Autodesk Inventor part; units mm, degrees
ref_plane "YZ Plane" through (0, 0, 0) normal (1, 0, 0) x (0, 1, 0)
ref_plane "XZ Plane" through (0, 0, 0) normal (0, 1, 0) x (-1, 0, 0)
ref_plane "XY Plane" through (0, 0, 0) normal (0, 0, 1) x (1, 0, 0)
sketch "스케치1" plane through (0, 0, 0) normal (0, 1, 0) x (-1, 0, 0)
  line L0 (-9.4, 28.75) -> (9.4, 28.75)
  line L1 (9.4, 28.75) -> (9.4, -28.75)
  line L2 (9.4, -28.75) -> (-9.4, -28.75)
  line L3 (-9.4, -28.75) -> (-9.4, 28.75)
  line L4 (-9.4, 28.75) -> (9.4, -28.75) construction
  line L5 (9.4, 28.75) -> (-9.4, -28.75) construction
  line L6 (-11.4, -30.75) -> (11.4, -30.75)
  line L7 (11.4, -30.75) -> (11.4, 30.75)
  line L8 (11.4, 30.75) -> (-11.4, 30.75)
  line L9 (-11.4, 30.75) -> (-11.4, -30.75)
  point P0 (0, 0)
  dimension "d0" = 18.8
  dimension "d1" = 57.5
  dimension "d2" = 2
extrude "돌출1" add sketch "스케치1" against normal blind 2 contours L0 L1 L2 L3
extrude "돌출2" add sketch "스케치1" against normal blind 6
sketch "스케치2" plane through (0, -6, 0) normal (0, -1, 0) x (1, 0, 0)
  line L0 (11.4, -30.75) -> (11.4, 30.75)
  line L1 (9.4, 28.75) -> (9.4, -28.75)
  line L2 (9.4, -28.75) -> (-9.4, -28.75)
  line L3 (11.4, -28.75) -> (9.1, -28.75)
  line L4 (9.1, -28.75) -> (9.1, -23.75)
  line L5 (9.1, -23.75) -> (11.4, -23.75)
  line L6 (11.4, -23.75) -> (11.4, -28.75)
  line L7 (0, 0) -> (0, -17.1125) construction
  line L8 (0, 0) -> (-6.0193, 0) construction
  line L9 (-11.4, -28.75) -> (-9.1, -28.75)
  line L10 (-9.1, -28.75) -> (-9.1, -23.75)
  line L11 (-9.1, -23.75) -> (-11.4, -23.75)
  line L12 (11.4, 28.75) -> (9.1, 28.75)
  line L13 (9.1, 28.75) -> (9.1, 23.75)
  line L14 (9.1, 23.75) -> (11.4, 23.75)
  line L15 (-9.1, 28.75) -> (-9.1, 23.75)
  line L16 (-11.4, 28.75) -> (-9.1, 28.75)
  line L17 (-9.1, 23.75) -> (-11.4, 23.75)
  line L18 (-11.4, 30.75) -> (-11.4, -30.75)
  line L19 (-11.4, -28.75) -> (-11.4, -23.75)
  line L20 (-11.4, 23.75) -> (-11.4, 28.75)
  line L21 (11.4, 23.75) -> (11.4, 28.75)
  point P0 (-9.1, -28.75)
  dimension "d7" = 0.3
  dimension "d8" = 5
extrude "돌출3" add sketch "스케치2" along normal blind 2 contours L3 L1 L5 L0 | L18 L16 L15 L17 | L2 L9 L18 L11 L10 | L2 L4 L5 L1 | L14 L1 L12 L0 | L14 L13 L12 L1
sketch "스케치3" plane through (0, 0, 0) normal (0, 1, 0) x (1, 0, 0)
  line L0 (6.25, -23) -> (-6.25, -23)
  line L1 (-6.25, -23) -> (-6.25, 23)
  line L2 (-6.25, 23) -> (6.25, 23)
  line L3 (6.25, 23) -> (6.25, -23)
  line L4 (6.25, -23) -> (-6.25, 23) construction
  line L5 (-6.25, -23) -> (6.25, 23) construction
  line L6 (0, -23) -> (0, 23) construction
  line L7 (9.4, -23.75) -> (9.4, 23.75) construction
  line L8 (9.4, 0) -> (-6.25, 0) construction
  line L9 (-6.25, -23) -> (-9.25, -23)
  line L10 (-9.25, -23) -> (-9.25, -13)
  line L11 (-9.25, -13) -> (-6.25, -13)
  line L12 (-6.25, -13) -> (-6.25, -23)
  line L13 (6.25, -23) -> (9.25, -23)
  line L14 (9.25, -23) -> (9.25, -13)
  line L15 (9.25, -13) -> (6.25, -13)
  line L16 (6.25, -13) -> (6.25, -23)
  line L17 (-6.25, 23) -> (-9.25, 23)
  line L18 (-9.25, 23) -> (-9.25, 13)
  line L19 (-9.25, 13) -> (-6.25, 13)
  line L20 (-6.25, 13) -> (-6.25, 23)
  line L21 (9.25, 13) -> (6.25, 13)
  line L22 (6.25, 13) -> (6.25, 23)
  line L23 (9.25, 23) -> (9.25, 13)
  line L24 (6.25, 23) -> (9.25, 23)
  point P0 (0, 0)
  dimension "d12" = 46
  dimension "d13" = 3
  dimension "d14" = 10
  dimension "d15" = 9.25
extrude "돌출4" add sketch "스케치3" along normal blind 5 contours L3 L15 L14 L13 | L9 L10 L11 L1 | L3 L24 L23 L21 | L19 L18 L17 L1
properties part number "converter2" material "고무, 검은색"
Here's how the part is built. I have some questions about the finished solid (model axes, mm). A direction names the side the tool comes from. Coordinates: 2 decimals unless noted, no trailing zeros. Write each loop counter-clockwise with the first axis right and the second up, starting at its lowest first coordinate (ties: lowest second). Pieces come first, ordered by that corner, then holes. Notation, with made-up numbers: (77.25, 46.5) -> (106.25, 46.5) arc R30 ccw to (106.25, 76.5) -> close; hole circle Ø6 at (47, 3.25). An arc over 180 degrees is marked (long way). Use a Markdown table: item, result. Add a question column.
(1) I'm going to push flat-ended pins straight in: P1, Ø3, axis at x = -3, z = -23.5, coming from the -Y side; P2, Ø2, axis at x = -3, z = -30, coming from the -Y side; P3, Ø1.5, axis at y = 2, z = -19, coming from the +X side. Where does each tip first touch, or does it pass through?
(2) If we section it at A-A, the plane y = -3.75: Write out the boundary of the cut face in (x, z).
(3) If we section it at C-C, the plane z = 15: Write out the boundary of the cut face in (x, y).
(4) If we section it at D-D, the plane x = 4.5: Write out the boundary of the cut face in (y, z), and give its area (3 significant figures).
(5) Please list where these lines run through material, in increasing order: line 1 (X direction, y = -4.5, z = 20.5); line 2 (X direction, y = 2.25, z = -14.5); line 3 (Y direction, x = -9.5, z = 17).
(6) If we section it at B-B, the plane y = -6.75: Write out the boundary of the cut face in (x, z), and give its area (3 significant figures).
(7) For faces 5 (the flat face through (-8, 2, -13)), 6 (the flat face through (-9.1, -7, 26)), 7 (the flat face through (-10, -6, 0)), 8 (the flat face through (-9.25, 2, -18)), which set-ups out of +Z, -Z, +X, -X, +Y, -Y let a thin tool reach every point of the face, with its end or its side?
(8) We'd pull the mould along X, two halves only. Please class faces 1 (the flat face through (8, 5, -18)), 2 (the flat face through (6.25, 2, 18)), 3 (the flat face through (0, -4, 28.75)), 4 (the flat face through (-9.25, 2, 18)): +X half, -X half, draft (parallel to the pull), parting line (faces both ways), or undercut.
Outcome:
| question | item | result |
|---|---|---|
| 1 | P1 | stops at y = -2 |
| 1 | P2 | stops at y = -6 |
| 1 | P3 | stops at x = 9.25 |
| 2 | outline | (-11.4, -30.75) -> (11.4, -30.75) -> (11.4, 30.75) -> (-11.4, 30.75) -> close; hole (-9.4, -28.75) -> (9.4, -28.75) -> (9.4, 28.75) -> (-9.4, 28.75) -> close |
| 3 | outline | (-11.4, -6) -> (-9.4, -6) -> (-9.4, -2) -> (9.4, -2) -> (9.4, -6) -> (11.4, -6) -> (11.4, 0) -> (9.25, 0) -> (9.25, 5) -> (6.25, 5) -> (6.25, 0) -> (-6.25, 0) -> (-6.25, 5) -> (-9.25, 5) -> (-9.25, 0) -> (-11.4, 0) -> close |
| 4 | outline | (-6, -30.75) -> (0, -30.75) -> (0, 30.75) -> (-6, 30.75) -> (-6, 28.75) -> (-2, 28.75) -> (-2, -28.75) -> (-6, -28.75) -> close |
| 4 | area | 139 mm^2 |
| 5 | line 1 | x = -11.4 to -9.4, 9.4 to 11.4 |
| 5 | line 2 | x = -9.25 to -6.25, 6.25 to 9.25 |
| 5 | line 3 | y = -6 to 0 |
| 6 | outline | (-11.4, -28.75) -> (-9.1, -28.75) -> (-9.1, -23.75) -> (-11.4, -23.75) -> close; (-11.4, 23.75) -> (-9.1, 23.75) -> (-9.1, 28.75) -> (-11.4, 28.75) -> close; (9.1, -28.75) -> (11.4, -28.75) -> (11.4, -23.75) -> (9.1, -23.75) -> close; (9.1, 23.75) -> (11.4, 23.75) -> (11.4, 28.75) -> (9.1, 28.75) -> close |
| 6 | area | 46.0 mm^2 |
| 7 | face 5 | +X, -X, +Y |
| 7 | face 6 | +Z, -Z, -Y |
| 7 | face 7 | +X, -X, -Y |
| 7 | face 8 | +Z, -Z, -X, +Y |
| 8 | face 1 | draft |
| 8 | face 2 | undercut |
| 8 | face 3 | undercut |
| 8 | face 4 | -X half |
